Read the model definition and answer for the solid it produces. Units are mm, in the model's axes. Face numbers are marked on the shaded views. Give positions to 0.01 mm unless a question says otherwise; leave off trailing zeros. Order: outer loops, then holes, each group sorted by start corner. A loop starts at its lowest first (then second) coordinate and runs counter-clockwise, first axis right, second up. Notation, with made-up numbers: M 84,37 L 96,37 A17 cw 96,51 Z; hole C 34,-40 d4. An arc over 180 degrees is marked long. One line per item, written item: value.
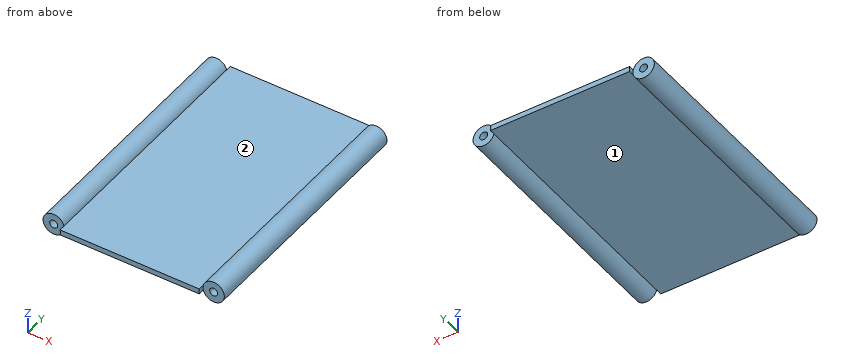
from build123d import *

# Parameters (mm, degrees)
SKETCH1_R           = 2.38125
BOSS_EXTRUDE1_DEPTH = 152.4
SKETCH2_R           = 6.35
CUT_EXTRUDE1_DEPTH  = 3.571875
SKETCH3_R           = 6.35
CUT_EXTRUDE3_DEPTH  = 3.175


with BuildPart() as part:
    # Sketch1 → Boss-Extrude1 (new body)
    with BuildSketch(Plane(origin=(0, 0, 0), x_dir=(1, 0, 0), z_dir=(0, 1, 0))):
        with BuildLine():
            Line((-41.476638938, 3.175), (0, 3.175))
            Line((0, 3.175), (0, 0))
            Line((0, 0), (-41.476638938, 0))
            ThreePointArc((-41.476638938, 0), (-53.975, 1.5875), (-41.476638938, 3.175))
        make_face()
        with Locations((-47.625, 1.5875)):
            Circle(SKETCH1_R, mode=Mode.SUBTRACT)
    boss_extrude1 = extrude(amount=BOSS_EXTRUDE1_DEPTH)

    # Sketch2 → Cut-Extrude1 (cut)
    with BuildSketch(Plane.XZ):
        with Locations((-47.625, -1.5875)):
            Circle(SKETCH2_R)
    cut_extrude1 = extrude(amount=-CUT_EXTRUDE1_DEPTH, mode=Mode.SUBTRACT)

    # Sketch3 → Cut-Extrude3 (cut)
    with BuildSketch(Plane(origin=(0, 152.4, 0), x_dir=(1, 0, 0), z_dir=(0, 1, 0))):
        with Locations((-47.625, 1.5875)):
            Circle(SKETCH3_R)
    cut_extrude3 = extrude(amount=-CUT_EXTRUDE3_DEPTH, mode=Mode.SUBTRACT)

    # Mirror2: Boss-Extrude1, Cut-Extrude1, Cut-Extrude3 across plane
    add(boss_extrude1.mirror(Plane(origin=(0, 152.4, -3.175), x_dir=(0, 0, 1), z_dir=(1, 0, 0))))
    add(cut_extrude1.mirror(Plane(origin=(0, 152.4, -3.175), x_dir=(0, 0, 1), z_dir=(1, 0, 0))), mode=Mode.SUBTRACT)
    add(cut_extrude3.mirror(Plane(origin=(0, 152.4, -3.175), x_dir=(0, 0, 1), z_dir=(1, 0, 0))), mode=Mode.SUBTRACT)


solid = part.part
1) Consider probe 1 along X at (y, z) = (63.5, -2.25); probe 2 along X at (y, z) = (70.5, -3); probe 3 along X at (y, z) = (143.5, 0.5). Determine where each line is inside the solid, lowest interval first.
Reported:
probe 1: x = -53.94 to -49.91, -45.34 to 45.34, 49.91 to 53.94
probe 2: x = -53.82 to -49.54, -45.71 to 45.71, 49.54 to 53.82
probe 3: x = -53.62 to -48.77, -46.48 to -41.63, 41.63 to 46.48, 48.77 to 53.62
2) Find section A-A, the plane z = 2.5. Write down the section's boundary in (x, y) (3 decimals), plus the area to 3 significant figures.
Reported:
outline: M -52.485,3.572 L -42.765,3.572 L -42.765,149.225 L -52.485,149.225 Z; M 42.765,3.572 L 52.485,3.572 L 52.485,149.225 L 42.765,149.225 Z
area: 2,830 mm^2
3) Determine the mould class of the marked faces 1 and 2 for opening direction X: +X half, -X half, draft (parallel to the pull), parting line (faces both ways), or undercut.
Reported:
face 1: undercut
face 2: undercut
4) Find section B-B, the plane y = 79.5. Count the separate pieces of the cut face and the enclosed holes in it, plus the area to 3 significant figures.
Reported:
separate pieces: 1
enclosed holes: 2
area: 480 mm^2
5) Find section C-C, the plane x = -11.5. Write down the section's boundary in (y, z) (3 decimals).
Reported:
outline: M 0,-3.175 L 152.4,-3.175 L 152.4,0 L 0,0 Z
6) Each of these flat-tipped pins is pushed along its axis until it touches: pin 1 Ø6 at (y, z) = (89.5, 3) entering from -X; pin 2 Ø4 at (x, z) = (-48.5, -2.5) entering from +Y (3 decimals); pin 3 Ø4.5 at (x, z) = (47.62, -1.59) entering from +Y; pin 4 Ø25 at (x, y) = (15.5, 82.5) entering from -Z (3 decimals). Where does it stop, or does it pass through?
Reported:
pin 1: stops at x = -53.77
pin 2: stops at y = 149.225
pin 3: passes through
pin 4: stops at z = -3.175
